The listing builds one solid part. Answer for the finished solid, in the listing's coordinates (mm). A direction names the side the tool comes from. Give positions to 0.01 mm unless a question says otherwise; leave off trailing zeros. Order: outer loops, then holes, each group sorted by start corner. A loop starts at its lowest first (then second) coordinate and runs counter-clockwise, first axis right, second up. Notation, with made-up numbers: (-19.5, -14) - (-15.5, -14) arc R12 ccw to (-15.5, -1) - close; hole circle Ø8 at (-6.5, 2). An arc over 180 degrees is marked (long way). Use CSV: the item, a comma, the result in double quotes.
```python
from build123d import *

# Parameters (mm, degrees)
ESQUISSE1_R        = 7.5
ESQUISSE1_R_2      = 5.05
BOSS_EXTRU_1_DEPTH = 1
ESQUISSE2_R        = 7.5
ESQUISSE2_R_2      = 2.05
BOSS_EXTRU_2_DEPTH = 9
CHANFREIN1_SIZE    = 1


with BuildPart() as part:
    # Esquisse1 → Boss.-Extru.1 (new body)
    with BuildSketch(Plane.XY):
        Circle(ESQUISSE1_R)
        Circle(ESQUISSE1_R_2, mode=Mode.SUBTRACT)
    extrude(amount=BOSS_EXTRU_1_DEPTH)

    # Esquisse2 → Boss.-Extru.2 (add)
    with BuildSketch(Plane.XY.offset(1)):
        Circle(ESQUISSE2_R)
        Circle(ESQUISSE2_R_2, mode=Mode.SUBTRACT)
    extrude(amount=BOSS_EXTRU_2_DEPTH)

    # Chanfrein1
    chanfrein1_edges = [part.edges().sort_by_distance(p)[0] for p in [
        (-7.5, 0, 10),
    ]]
    chamfer(chanfrein1_edges, length=CHANFREIN1_SIZE)


solid = part.part
```
Item 1: The part is cut by section A-A (x = 0). Give the vertices of the cut face in (y, z).
Taken from the geometry:
outline,"(-7.5, 0) - (-5.05, 0) - (-5.05, 1) - (-2.05, 1) - (-2.05, 10) - (-6.5, 10) - (-7.5, 9) - close; (2.05, 1) - (5.05, 1) - (5.05, 0) - (7.5, 0) - (7.5, 9) - (6.5, 10) - (2.05, 10) - close"
Item 2: The part is cut by section B-B (z = 4). Give the vertices of the cut face in (x, y), and give its area (3 significant figures).
Taken from the geometry:
outline,"circle Ø15 at (0, 0); hole circle Ø4.1 at (0, 0)"
area,"164 mm^2"
Item 3: Which of the six approach directions +Z, -Z, +X, -X, +Y, -Y give full straight-line access (tool end or side, diameter ignored) to faces 1 (the face through (-2, 2, 10)), 2 (the face through (4.817, 1.517, 0.493))?
Taken from the geometry:
face 1,"+Z, +X, -X, +Y, -Y"
face 2,"-Z"
Item 4: The mould has two halves that part along Y. Classify faces 3 (the face through (-0.267, 2.033, 5.437)), 4 (the face through (2, -5, 0)), 5 (the face through (-7.493, 0.33, 4.437)): +Y half, -Y half, draft (parallel to the pull), parting line (faces both ways), or undercut.
Taken from the geometry:
face 3,"undercut"
face 4,"draft"
face 5,"parting line"
Item 5: Find the intervals of material crossed by line 1 along Y through (x, z) = (0, 8); line 2 along Y through (x, z) = (0, 0.5); line 3 along Z through (x, y) = (4.25, -2), in increasing order.
Taken from the geometry:
line 1,"-7.5 to -2.05, 2.05 to 7.5"
line 2,"-7.5 to -5.05, 5.05 to 7.5"
line 3,"1 to 10"
Item 6: Each of these flat-tipped pins is pushed along its axis until it touches: pin 1 (3 mm diameter, centred on y = -4, z = 2, fed in from +X); pin 2 (2 mm diameter, centred on x = 3.5, z = 3, fed in from -Y); pin 3 (1 mm diameter, centred on x = -5, z = 5, fed in from -Y). Where does it stop, or does it pass through?
Taken from the geometry:
pin 1,"x = 7.07"
pin 2,"y = -7.07"
pin 3,"y = -6"
